Geometry check sheet. Reference: drawing and pictorial views, mm from the part's lowest x, y, z. A direction names the side the tool comes from. Round coordinates to 2 decimals unless told otherwise and drop trailing zeros. Loops run counter-clockwise (first coordinate to the right, second up) from the corner with the lowest first, then second, coordinate; pieces in that order, holes last. Notation, with made-up numbers: (73, -18) -> (91, -18) arc R26 ccw to (91, 16) -> close; hole circle Ø8 at (45.25, 18). An arc over 180 degrees is marked (long way). Use one line per item in the form item = value.
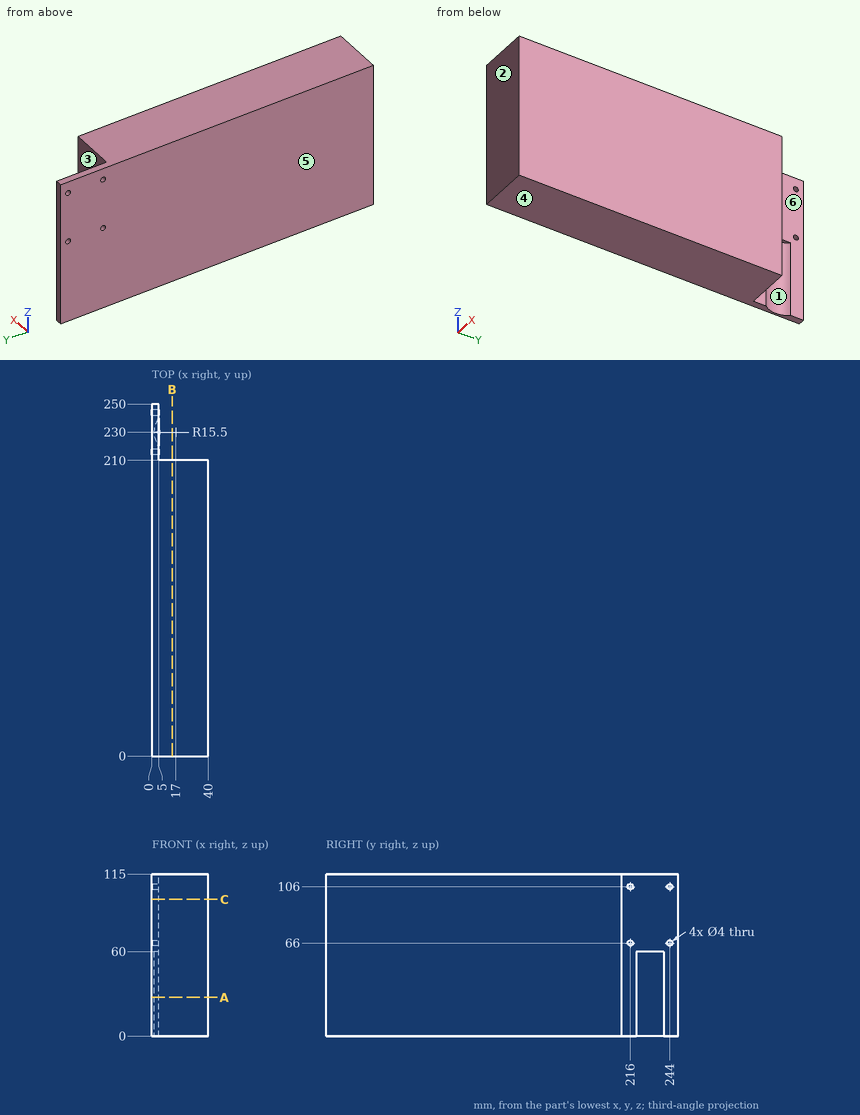
1. Section check B-B (x = 14.5). Record the boundary of the cut face in (y, z), then the cut area to 4 significant figures.
Return value:
outline = (0, 0) -> (210, 0) -> (210, 115) -> (0, 115) -> close
area = 24,150 mm2
2. Section check C-C (z = 97). Record the boundary of the cut face in (x, y), then the cut area to 3 significant figures.
Return value:
outline = (0, 0) -> (40, 0) -> (40, 210) -> (5, 210) -> (5, 250) -> (0, 250) -> close
area = 8,600 mm2
3. Gauge pin test, flat ends, axial feed: pin 1 (3.5 mm diameter, centred on y = 216, z = 66, fed in from -X); pin 2 (6.5 mm diameter, centred on y = 244, z = 106, fed in from +X); pin 3 (6 mm diameter, centred on x = 15, z = 55.5, fed in from +Y); pin 4 (1.8 mm diameter, centred on x = 3.5, y = 226, fed in from -Z). Record the tip position at first contact, or that the pin passes through.
Return value:
pin_1 = through
pin_2 = 5
pin_3 = 210
pin_4 = 60
4. Tool access check on the marked faces 5 and 6. Record the directions out of +Z, -Z, +X, -X, +Y, -Y that give a thin tool (end or side, any length) a straight path to the whole face; none if there is none.
Return value:
face_5 = +Z, -Z, -X, +Y, -Y
face_6 = +Z, -Z, +X, +Y
5. Material ranges on line 1 along Z through (x, y) = (1.7, 216); line 2 along Y through (x, z) = (20.5, 25); line 3 along X through (y, z) = (214, 50.5), recorded low to high.
Return value:
line_1 = 0 to 64, 68 to 104, 108 to 115
line_2 = 0 to 210
line_3 = 0 to 5
6. Section check A-A (z = 27.5). Record the boundary of the cut face in (x, y).
Return value:
outline = (0, 0) -> (40, 0) -> (40, 210) -> (5, 210) -> (5, 220.19) arc R15.5 cw to (5, 239.81) -> (5, 250) -> (0, 250) -> close
7. Mould release check, pull along Y, two halves, no side actions. Record for the marked faces 1, 2, 3 and 4: released by +Y, released by -Y, zero draft, split by the parting line, or undercut.
Return value:
face_1 = undercut
face_2 = released by -Y
face_3 = released by +Y
face_4 = zero draft
